```python
from build123d import *

# Parameters (mm, degrees)
F0_W     = 50.8
F0_H     = 50.8
F1_DEPTH = 50.8
F2_W     = 40.64
F2_H     = 40.64
F3_DEPTH = 49.53
F4_W     = 7.850907743
F4_H     = 21.4745448902
F5_DEPTH = 25.4
F6_W     = 12.7
F6_H     = 12.7
F7_DEPTH = 7.62
F8_W     = 35.329092294
F8_H     = 8.312728256
F9_DEPTH = 50.8


with BuildPart() as f1:
    # F0 (on Top) → F1 (new body)
    with BuildSketch(Plane.XY):
        with Locations((2.078182064, 0.7973827244)):
            Rectangle(F0_W, F0_H)
    extrude(amount=F1_DEPTH)

    # F2 (on face) → F3 (cut)
    with BuildSketch(Plane.XY.offset(50.8)):
        with Locations((1.8472736701, 1.0047121724)):
            Rectangle(F2_W, F2_H)
    extrude(amount=-F3_DEPTH, mode=Mode.SUBTRACT)

    # F4 (on face) → F5 (cut)
    with BuildSketch(Plane.XZ.offset(24.6026172756)):
        with Locations((-12.8154549748, 13.0454613827)):
            Rectangle(F4_W, F4_H)
    extrude(amount=-F5_DEPTH, mode=Mode.SUBTRACT)

    # F6 (on face) → F7 (cut)
    with BuildSketch(Plane.XZ.offset(24.6026172756)):
        with Locations((11.8126636371, 35.6554915783)):
            Rectangle(F6_W, F6_H)
    extrude(amount=-F7_DEPTH, mode=Mode.SUBTRACT)

    # F8 (on face) → F9 (cut)
    with BuildSketch(Plane(origin=(-23.321817936, 0, 0), x_dir=(0, -1, 0), z_dir=(-1, 0, 0))):
        with Locations((0, 36.7136429995)):
            Rectangle(F8_W, F8_H)
    extrude(amount=-F9_DEPTH, mode=Mode.SUBTRACT)


solid = f1.part
```
For this review, take the finished solid that the model builds, in its own axes (mm). A direction names the side the tool comes from. Coordinates: 2 decimals unless noted, no trailing zeros. Loops run counter-clockwise (first coordinate to the right, second up) from the corner with the lowest first, then second, coordinate; pieces in that order, holes last.
1. For faces 1 (the flat face through (-21, 0, 40.87)), 2 (the flat face through (2, 1, 0)), 3 (the flat face through (22.167, 1, 26)), 4 (the flat face through (18.163, -22, 36)), 5 (the flat face through (27.478, 0, 25)), list the 3-axis set-ups (+Z, -Z, +X, -X, +Y, -Y) from which the entire face can be reached by the end or side of a thin tool; tool diameter is ignored.
2. Add section B-B, the plane x = 9. Give the boundary of the cut face in (y, z), then the cut area to 3 significant figures.
3. For line 1 (X direction, y = 2.5, z = 7); line 2 (Z direction, x = 9, y = -21); line 3 (Y direction, x = -3, z = 11.5), list the stretches that pass through material, from the lowest coordinate up.
4. Add section D-D, the plane x = -8. Give the boundary of the cut face in (y, z), then the cut area to 3 significant figures.
5. Add section C-C, the plane z = 36. Give the boundary of the cut face in (x, y), then the cut area to 3 significant figures.
6. Add section A-A, the plane y = -6. Give the boundary of the cut face in (x, z), then the cut area to 3 significant figures.
7. Insertion check: P1, Ø1.5, axis at x = -13.5, y = 0.5, coming from the +Z side; P2, Ø2.5, axis at x = -13.5, y = -21.5, coming from the -Z side. Each pin has a flat end and moves straight along its axis. Give the tip position at first contact, or say it passes through.
8. Mouldability with a two-part tool opening along Z and no side actions: class faces 6 (the flat face through (-21, 1, 50.8)), 7 (the flat face through (-21, 0, 32.557)), 8 (the flat face through (-23.322, 0, 25)), 9 (the flat face through (25, 0, 40.87)) as +Z half, -Z half, draft (parallel to the pull), parting line (faces both ways), or undercut.
Result:
1. face 1: +X, -X
1. face 2: -Z, +X, -X, +Y, -Y
1. face 3: +Z
1. face 4: -Y
1. face 5: +Z, -Z, +X, +Y, -Y
2. outline: (-24.6, 0) - (26.2, 0) - (26.2, 50.8) - (21.32, 50.8) - (21.32, 1.27) - (-19.32, 1.27) - (-19.32, 29.31) - (-24.6, 29.31) - close; (-24.6, 42.01) - (-19.32, 42.01) - (-19.32, 50.8) - (-24.6, 50.8) - close
2. area: 501 mm2
3. line 1: x = -23.32 to -18.47, 22.17 to 27.48
3. line 2: z = 0 to 29.31, 42.01 to 50.8
3. line 3: y = -24.6 to -19.32, 21.32 to 26.2
4. outline: (-24.6, 0) - (26.2, 0) - (26.2, 50.8) - (21.32, 50.8) - (21.32, 1.27) - (-19.32, 1.27) - (-19.32, 50.8) - (-24.6, 50.8) - close
4. area: 568 mm2
5. outline: (-23.32, -24.6) - (5.46, -24.6) - (5.46, -19.32) - (-18.47, -19.32) - (-18.47, -17.66) - (-23.32, -17.66) - close; (-23.32, 17.66) - (-18.47, 17.66) - (-18.47, 21.32) - (22.17, 21.32) - (22.17, 17.66) - (27.48, 17.66) - (27.48, 26.2) - (-23.32, 26.2) - close; (18.16, -24.6) - (27.48, -24.6) - (27.48, -17.66) - (22.17, -17.66) - (22.17, -19.32) - (18.16, -19.32) - close
5. area: 503 mm2
6. outline: (-23.32, 0) - (27.48, 0) - (27.48, 32.56) - (22.17, 32.56) - (22.17, 1.27) - (-18.47, 1.27) - (-18.47, 32.56) - (-23.32, 32.56) - close; (-23.32, 40.87) - (-18.47, 40.87) - (-18.47, 50.8) - (-23.32, 50.8) - close; (22.17, 40.87) - (27.48, 40.87) - (27.48, 50.8) - (22.17, 50.8) - close
6. area: 483 mm2
7. P1: stops at z = 1.27
7. P2: stops at z = 0
8. face 6: +Z half
8. face 7: undercut
8. face 8: draft
8. face 9: undercut
